Input: part model. Units: mm. Frame: model coordinates. Face numbers are marked on the shaded views. A direction names the side the tool comes from. Coordinates: 2 decimals unless noted, no trailing zeros. Order: outer loops, then holes, each group sorted by start corner. A loop starts at its lowest first (then second) coordinate and runs counter-clockwise, first axis right, second up. Notation, with made-up numbers: (89.25, -2) -> (96.25, -2) arc R19 ccw to (96.25, 12) -> close; hole circle Ø4 at (17, 87). An arc over 180 degrees is marked (long way). One line per item, written item: value. Start each with the question number.
from build123d import *

# Parameters (mm, degrees)
SKETCH1_W                    = 312
SKETCH1_H                    = 200
BASE_FLANGE1_DEPTH           = 6
EDGE_FLANGE1_STRIP_W         = 44
EDGE_FLANGE1_STRIP_H         = 6
EDGE_FLANGE1_STRIP_CUT_DEPTH = 200
EDGE_FLANGE1_DEPTH           = 200
EDGE_FLANGE2_STRIP_W         = 44
EDGE_FLANGE2_STRIP_H         = 6
EDGE_FLANGE2_STRIP_CUT_DEPTH = 200
EDGE_FLANGE2_DEPTH           = 200
SKETCH24_R                   = 45
CUT_EXTRUDE1_DEPTH           = 10
SKETCH27_R                   = 11
CUT_EXTRUDE4_DEPTH           = 10
SKETCH28_R                   = 9
CUT_EXTRUDE5_DEPTH           = 445.234172481


# Sheet-metal steps are written as plain solids
with BuildPart() as part:
    # Sketch1 → Base-Flange1 (new body)
    with BuildSketch(Plane.XY):
        Rectangle(SKETCH1_W, SKETCH1_H)
    extrude(amount=-BASE_FLANGE1_DEPTH)

    # Edge-Flange1 strip (across the edge) → Edge-Flange1 strip cut (cut)
    with BuildSketch(Plane(origin=(-156, -100, -6), x_dir=(1, 0, 0), z_dir=(0, 1, 0))):
        with Locations((-6, -3)):
            Rectangle(EDGE_FLANGE1_STRIP_W, EDGE_FLANGE1_STRIP_H)
    extrude(amount=EDGE_FLANGE1_STRIP_CUT_DEPTH, mode=Mode.SUBTRACT)

    # Edge-Flange1 section (across the edge) → Edge-Flange1 (add)
    with BuildSketch(Plane(origin=(-156, -100, -6), x_dir=(1, 0, 0), z_dir=(0, 1, 0))):
        with BuildLine():
            Line((0, 10), (0, 294))
            Line((0, 294), (6, 294))
            Line((6, 294), (6, 10))
            ThreePointArc((6, 10), (8.928932188, 2.928932188), (16, 0))
            Line((16, 0), (16, -6))
            ThreePointArc((16, -6), (4.686291501, -1.313708499), (0, 10))
        make_face()
    extrude(amount=EDGE_FLANGE1_DEPTH)

    # Edge-Flange2 strip (across the edge) → Edge-Flange2 strip cut (cut)
    with BuildSketch(Plane(origin=(156, 100, -6), x_dir=(-1, 0, 0), z_dir=(0, -1, 0))):
        with Locations((-6, -3)):
            Rectangle(EDGE_FLANGE2_STRIP_W, EDGE_FLANGE2_STRIP_H)
    extrude(amount=EDGE_FLANGE2_STRIP_CUT_DEPTH, mode=Mode.SUBTRACT)

    # Edge-Flange2 section (across the edge) → Edge-Flange2 (add)
    with BuildSketch(Plane(origin=(156, 100, -6), x_dir=(-1, 0, 0), z_dir=(0, -1, 0))):
        with BuildLine():
            Line((0, 10), (0, 294))
            Line((0, 294), (6, 294))
            Line((6, 294), (6, 10))
            ThreePointArc((6, 10), (8.928932188, 2.928932188), (16, 0))
            Line((16, 0), (16, -6))
            ThreePointArc((16, -6), (4.686291501, -1.313708499), (0, 10))
        make_face()
    extrude(amount=EDGE_FLANGE2_DEPTH)

    # Sketch24 → Cut-Extrude1 (cut)
    with BuildSketch(Plane.XY):
        Circle(SKETCH24_R)
    extrude(amount=-CUT_EXTRUDE1_DEPTH, mode=Mode.SUBTRACT)

    # Sketch27 → Cut-Extrude4 (cut)
    with BuildSketch(Plane.XY):
        with Locations((58.35, 58.35)):
            Circle(SKETCH27_R)
        with Locations((58.35, -58.35)):
            Circle(SKETCH27_R)
        with Locations((-58.35, -58.35)):
            Circle(SKETCH27_R)
        with Locations((-58.35, 58.35)):
            Circle(SKETCH27_R)
    extrude(amount=-CUT_EXTRUDE4_DEPTH, mode=Mode.SUBTRACT)

    # Sketch28 → Cut-Extrude5 (cut, through all)
    with BuildSketch(Plane.ZY.offset(156)):
        with Locations((-270, 60)):
            Circle(SKETCH28_R)
        with Locations((-270, -60)):
            Circle(SKETCH28_R)
    extrude(amount=-CUT_EXTRUDE5_DEPTH, mode=Mode.SUBTRACT)


solid = part.part
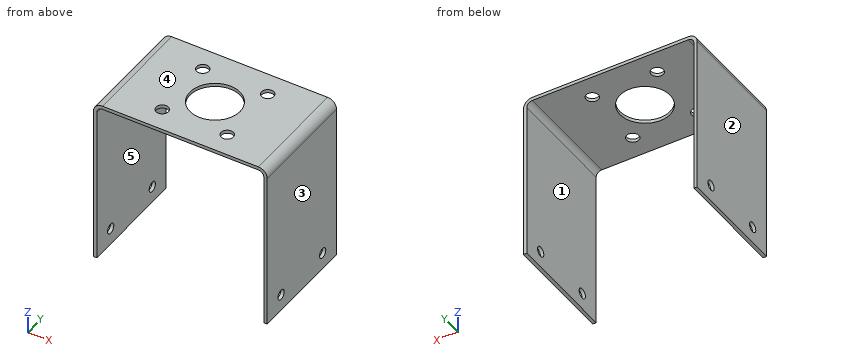
1) Section query D-D, the plane x = 0. Return the cut outline in (y, z), plus the area to 3 significant figures.
2) Access query for the marked faces 4 and 5. Directions: +Z, -Z, +X, -X, +Y, -Y. A direction counts if a zero-diameter tool reaches every point of the face in a straight line with its end or side. Return the directions, or none.
3) Section query A-A, the plane z = -162.5. Return the cut outline in (x, y).
4) Ray query, line 1 along Y through (x, z) = (58, -1); line 2 along Y through (x, z) = (153, -270); line 3 along X through (y, z) = (71.5, -69.5). Return the intervals inside material, ascending. Write a range as from..to.
5) Section query C-C, the plane x = -58.35. Return the cut outline in (y, z), plus the area to 3 significant figures.
6) Section query B-B, the plane y = 0. Return the cut outline in (x, z).
7) Mould query, pull axis X, two halves, no side actions, for the marked faces 1, 2 and 3. Classes: +X half, -X half, draft (parallel to the pull), parting line (faces both ways), or undercut.
Entries:
1. outline: (-100, -6) -> (-45, -6) -> (-45, 0) -> (-100, 0) -> close; (45, -6) -> (100, -6) -> (100, 0) -> (45, 0) -> close
1. area: 660 mm2
2. face 4: +Z, +X, -X, +Y, -Y
2. face 5: -Z, +Y, -Y
3. outline: (-156, -100) -> (-150, -100) -> (-150, 100) -> (-156, 100) -> close; (150, -100) -> (156, -100) -> (156, 100) -> (150, 100) -> close
4. line 1: y = -100..-69.34, -47.36..47.36, 69.34..100
4. line 2: y = -100..-69, -51..51, 69..100
4. line 3: x = -156..-150, 150..156
5. outline: (-100, -6) -> (-69.35, -6) -> (-69.35, 0) -> (-100, 0) -> close; (-47.35, -6) -> (47.35, -6) -> (47.35, 0) -> (-47.35, 0) -> close; (69.35, -6) -> (100, -6) -> (100, 0) -> (69.35, 0) -> close
5. area: 936 mm2
6. outline: (-156, -300) -> (-150, -300) -> (-150, -16) arc R10 cw to (-140, -6) -> (-45, -6) -> (-45, 0) -> (-140, 0) arc R16 ccw to (-156, -16) -> close; (45, -6) -> (140, -6) arc R10 cw to (150, -16) -> (150, -300) -> (156, -300) -> (156, -16) arc R16 ccw to (140, 0) -> (45, 0) -> close
7. face 1: undercut
7. face 2: -X half
7. face 3: +X half
